Part model, mm, in its own coordinate system. A direction names the side the tool comes from. Round coordinates to 2 decimals unless told otherwise and drop trailing zeros. Write each loop counter-clockwise with the first axis right and the second up, starting at its lowest first coordinate (ties: lowest second). Pieces come first, ordered by that corner, then holes. Notation, with made-up numbers: (-16.75, -20) -> (1.25, -20) arc R30 ccw to (1.25, 5) -> close; hole circle Ø10 at (-14, 61.5). An arc over 180 degrees is marked (long way). Use CSV: the item, a comma, the result in double quotes. Start each with the question number.
(1) Two-plate mould, pull along X, no slides. Class faces 4 (the flat face through (-0.51, -0.86, 6.63)), 5 (the cylindrical face through (-0.05, 1.25, -0.94)), 6 (the flat face through (0, 0, -7.25)), 7 (the flat face through (1, 0, 7)): released by +X, released by -X, zero draft, split by the parting line, or undercut.
(2) Drop flat-ended pins along their axis: pin 1 (1.6 mm diameter, centred on x = -0.5, y = 0, fed in from +Z); pin 2 (1.5 mm diameter, centred on x = 1, z = -0.5, fed in from -Y). Give the stop position or say it passes through.
(3) Saw through at B-B (z = -5.75). Give the cut face in (x, y), plus the area to 3 significant figures.
(4) Probe line 1 (Y direction, x = 0.1, z = -3.75); line 2 (Y direction, x = -0.75, z = -5); line 3 (Z direction, x = -1.35, y = -1.2). List the from-to ranges inside material, lowest first. Write a range as [from, to].
(5) Which spindle directions (+Z, -Z, +X, -X, +Y, -Y) get a long thin tool onto all of the face, cutting with end or side? Do faces 1 (the flat face through (0.51, 0.86, 6.63)), 2 (the cylindrical face through (-1.52, 1.66, 6.01)), 3 (the flat face through (1, 1, 4.75)). Say none if no direction does.
```python
from build123d import *

# Parameters (mm, degrees)
CUT_EXTRUDE1_DEPTH = 1.25


with BuildPart() as part:
    # Sketch3 → Revolve1 (revolve)
    with BuildSketch(Plane(origin=(0, 0, 0), x_dir=(0, 0, -1), z_dir=(1, 0, 0)), mode=Mode.PRIVATE) as revolve1_sk:
        with BuildLine():
            Line((-7.25, 2.063775365), (-7.25, 1))
            Line((-7.25, 1), (-6, 1))
            Line((-6, 1), (-6, 0))
            Line((-6, 0), (7.25, 0))
            Line((7.25, 0), (7.25, 0.795336663))
            Line((7.25, 0.795336663), (6.795336663, 1.25))
            Line((6.795336663, 1.25), (-4.75, 1.25))
            Line((-4.75, 1.25), (-4.75, 2.063775365))
            ThreePointArc((-4.75, 2.063775365), (-4.753211332, 2.079919823), (-4.762356433, 2.093606433))
            Line((-4.762356433, 2.093606433), (-4.906393567, 2.237643567))
            ThreePointArc((-4.906393567, 2.237643567), (-4.920080177, 2.246788668), (-4.936224635, 2.25))
            Line((-4.936224635, 2.25), (-7.063775365, 2.25))
            ThreePointArc((-7.063775365, 2.25), (-7.079919823, 2.246788668), (-7.093606433, 2.237643567))
            Line((-7.093606433, 2.237643567), (-7.237643567, 2.093606433))
            ThreePointArc((-7.237643567, 2.093606433), (-7.246788668, 2.079919823), (-7.25, 2.063775365))
        make_face()
    revolve(revolve1_sk.sketch.rotate(Axis((0, 0, 7.25), (0, 0, -1)), 180), axis=Axis((0, 0, 7.25), (0, 0, -1)))

    # Sketch4 → Cut-Extrude1 (cut)
    with BuildSketch(Plane.XY.offset(7.25)):
        Polygon((0, 1.154700538), (-1, 0.577350269), (-1, -0.577350269), (0, -1.154700538), (1, -0.577350269), (1, 0.577350269), align=None)
    extrude(amount=-CUT_EXTRUDE1_DEPTH, mode=Mode.SUBTRACT)


solid = part.part
```
Answers:
1,face 4,"undercut"
1,face 5,"split by the parting line"
1,face 6,"zero draft"
1,face 7,"undercut"
2,pin 1,"stops at z = 7.25"
2,pin 2,"stops at y = -1.22"
3,outline,"circle Ø2.5 at (0, 0)"
3,area,"4.91 mm²"
4,line 1,"y = [-1.25, 1.25]"
4,line 2,"y = [-1, 1]"
4,line 3,"z = [4.75, 7.25]"
5,face 1,"+Z"
5,face 2,"+Z, -Z"
5,face 3,"-Z"
